Part model, mm, in its own coordinate system. Round coordinates to 2 decimals unless told otherwise and drop trailing zeros. Write each loop counter-clockwise with the first axis right and the second up, starting at its lowest first coordinate (ties: lowest second). Pieces come first, ordered by that corner, then holes. Notation, with made-up numbers: (10, 10) -> (27, 10) arc R32 cw to (27, 44) -> close; hole circle Ø1 at (6, -15.75). An arc over 180 degrees is marked (long way). Return JSON: item names as keys, results as strings. Group by question number.
(1) Mould opens along Y. For faces 1 (the cylindrical face through (5.916, -88.738, 15.021)), 2 (the cylindrical face through (5.89, 18.146, -55.642)), 3 (the cylindrical face through (5.9, 65.9, -13.4)) say: +Y half, -Y half, draft (parallel to the pull), parting line (faces both ways), or undercut.
(2) Saw through at A-A (z = 0). List the corners of the cut face in (x, y), plus the area to 3 significant figures.
(3) Drill centre lines: L1, parallel to Y at x = 5.25, z = 0; L2, parallel to Z at x = 5.75, y = 0; L3, parallel to Z at x = 4, y = -24. Where is each one in solid material? Low to high. Write a range as from..to.
(4) Saw through at B-B (y = 0). List the corners of the cut face in (x, z), plus the area to 3 significant figures.
(5) Saw through at C-C (y = -58). List the corners of the cut face in (x, z).
(6) Drop flat-ended pins along their axis: pin 1 Ø1.5 at (x, y) = (5, -66.5) entering from +Z; pin 2 Ø2 at (x, y) = (5.5, -51) entering from -Z; pin 3 Ø4 at (x, z) = (7, -12.5) entering from +Y. Give the stop position or say it passes through.
from build123d import *

# Parameters (mm, degrees)
SKETCH_1_R               = 67.25
EXTRUDE_1_DEPTH          = 12
EXTRUDE_2_DEPTH          = 12
CUT_EXTRUDE_1_DEPTH      = 113.989214087
CUT_EXTRUDE_1_DEPTH_BACK = 113.989214087
SKETCH_3_R               = 50


with BuildPart() as part:
    # ｽｹｯﾁ1 → ﾎﾞｽ - 押し出し1 (new body)
    with BuildSketch(Plane(origin=(0, 0, 0), x_dir=(0, 0, -1), z_dir=(1, 0, 0))):
        Circle(SKETCH_1_R)
    extrude(amount=EXTRUDE_1_DEPTH)

    # ｽｹｯﾁ2 → ﾎﾞｽ - 押し出し2 (add)
    with BuildSketch(Plane(origin=(0, 0, 0), x_dir=(0, 0, -1), z_dir=(1, 0, 0))):
        with BuildLine():
            Line((-41.549382629, -52.879214282), (-38.758443712, -81.226738461))
            ThreePointArc((-38.758443712, -81.226738461), (-14.671715608, -88.796062757), (10.569667713, -89.37719018))
            Line((10.569667713, -89.37719018), (22.328272087, -63.435090964))
            Line((22.328272087, -63.435090964), (-41.549382629, -52.879214282))
        make_face()
    extrude(amount=EXTRUDE_2_DEPTH)

    # ｽｹｯﾁ3 → ｶｯﾄ - 押し出し1 (cut, two sides: drawn at the far end of the back side and taken through both)
    with BuildSketch(Plane(origin=(0, 0, 0), x_dir=(0, 0, -1), z_dir=(1, 0, 0)).offset(-CUT_EXTRUDE_1_DEPTH_BACK)):
        Circle(SKETCH_3_R)
    extrude(amount=CUT_EXTRUDE_1_DEPTH + CUT_EXTRUDE_1_DEPTH_BACK, mode=Mode.SUBTRACT)

    # ｽｹｯﾁ4 → ｶｯﾄ - 回転1 (revolve, cut)
    with BuildSketch(Plane(origin=(6, 0, 0), x_dir=(0, 0, -1), z_dir=(1, 0, 0)), mode=Mode.PRIVATE) as cut_revolve_1_sk:
        Polygon((-44.399328848, 7.328000946), (-73.998881413, 12.21333491), (-74.405992577, 9.74670553), (-44.806440011, 4.861371566), align=None)
    revolve(cut_revolve_1_sk.sketch.rotate(Axis((6, 0, 0), (0, 0.1628444654719115, 0.9866517521725523)), 180), axis=Axis((6, 0, 0), (0, 0.1628444654719115, 0.9866517521725523)), mode=Mode.SUBTRACT)

    # ｽｹｯﾁ5 → ｶｯﾄ - 回転2 (revolve, cut)
    with BuildSketch(Plane(origin=(6, 0, 0), x_dir=(0, 0, -1), z_dir=(1, 0, 0)), mode=Mode.PRIVATE) as cut_revolve_2_sk:
        Polygon((43.338895176, 12.113635497), (72.231491959, 20.189392495), (71.55851221, 22.597108894), (42.665915426, 14.521351896), align=None)
    revolve(cut_revolve_2_sk.sketch.rotate(Axis((6, 0, 0), (0, 0.2691918999319745, -0.9630865594592284)), 180), axis=Axis((6, 0, 0), (0, 0.2691918999319745, -0.9630865594592284)), mode=Mode.SUBTRACT)


solid = part.part
Computed values:
{
 "1": {"face 1": "-Y half", "face 2": "undercut", "face 3": "parting line"},
 "2": {"outline": "(0, -90) -> (12, -90) -> (12, -50) -> (0, -50) -> close; (0, 50) -> (12, 50) -> (12, 67.25) -> (0, 67.25) -> close", "area": "687 mm2"},
 "3": {"L1": "-90..-50, 50..67.25", "L2": "-67.25..-50, 50..67.25", "L3": "-62.82..-43.86, 43.86..62.82"},
 "4": {"outline": "(0, -67.25) -> (12, -67.25) -> (12, -50) -> (0, -50) -> close; (0, 50) -> (12, 50) -> (12, 67.25) -> (0, 67.25) -> close", "area": "414 mm2"},
 "5": {"outline": "(0, -34.04) -> (12, -34.04) -> (12, 41.05) -> (0, 41.05) -> close"},
 "6": {"pin 1": "z = 40.28", "pin 2": "z = -44.97", "pin 3": "y = 66.43"}
}
